Autodesk Inventor part; units mm, degrees
ref_plane "YZ Plane" through (0, 0, 0) normal (1, 0, 0) x (0, 1, 0)
ref_plane "XZ Plane" through (0, 0, 0) normal (0, 1, 0) x (-1, 0, 0)
ref_plane "XY Plane" through (0, 0, 0) normal (0, 0, 1) x (1, 0, 0)
sketch "Sketch1" plane through (0, 0, 0) normal (0, 0, 1) x (1, 0, 0)
  line L0 (-212.5, -81.5) -> (212.5, -81.5)
  line L1 (212.5, -81.5) -> (212.5, 81.5)
  line L2 (212.5, 81.5) -> (-212.5, 81.5)
  line L3 (-212.5, 81.5) -> (-212.5, -81.5)
  line L4 (-212.5, -81.5) -> (212.5, 81.5) construction
  line L5 (212.5, -81.5) -> (-212.5, 81.5) construction
  point P0 (0, 0)
  dimension "d0" = 163
  dimension "d1" = 425
extrude "Extrusion1" add sketch "Sketch1" against normal blind 335
sketch "Sketch2" plane through (-212.5, -81.5, 0) normal (0, -1, 0) x (1, 0, 0)
  line L0 (0, 0) -> (425, 0) construction
  line L1 (425, -8) -> (409.5, -8)
  line L2 (409.5, -8) -> (409.5, -28)
  line L3 (409.5, -28) -> (425, -28)
  line L4 (425, -28) -> (425, -8)
  line L5 (20, -10) -> (0, -10)
  line L6 (0, -10) -> (0, -25.5)
  line L7 (0, -25.5) -> (20, -25.5)
  line L8 (20, -25.5) -> (20, -10)
  line L9 (0, -10) -> (0, 0) construction
  line L10 (425, -8) -> (425, 0) construction
  point P0 (212.5, 0)
  dimension "d0" = 163
  dimension "d4" = 8
  dimension "d5" = 10
  dimension "d6" = 15.5
  dimension "d7" = 20
  dimension "d8" = 15.5
  dimension "d9" = 20
extrude "Extrusion2" add sketch "Sketch2" along normal blind 6
sketch "Sketch3" plane through (212.5, -81.5, 0) normal (1, 0, 0) x (0, 0, -1)
  line L0 (0, 0) -> (0, 163)
  line L1 (0, 0) -> (-5, 0)
  line L2 (-5, 0) -> (-40, 47)
  line L3 (-40, 47) -> (-90, 47)
  line L4 (-90, 47) -> (-90, 87)
  line L5 (-90, 87) -> (-69, 87)
  line L6 (-69, 93) -> (-34.909, 105.3518)
  line L7 (-69, 87) -> (-69, 93)
  arc A0 (-34.909, 105.3518) -> (-5, 148) centre (-50.3612, 148) ccw
  line L8 (-34.909, 105.3518) -> (0, 118) construction
  arc A1 (-37.8496, 44.1124) -> (-43.6003, 47) centre (-43.6003, 39.8299) ccw
  line L9 (-5, 148) -> (-5, 163)
  line L10 (-5, 163) -> (0, 163)
  dimension "d12" = 5
  dimension "d13" = 47
  dimension "d14" = 35
  dimension "d15" = 40
  dimension "d16" = 90
  dimension "d17" = 118
  dimension "d18" = 93
  dimension "d19" = 69
  dimension "d23" = 55
  dimension "d26" = 5
  dimension "d27" = 15
extrude "Extrusion3" add sketch "Sketch3" against normal blind 35
sketch "Sketch4" plane through (-212.5, -81.5, 0) normal (-1, 0, 0) x (0, 0, 1)
  line L0 (0, 0) -> (0, 163)
  line L1 (0, 0) -> (5, 0)
  line L2 (5, 0) -> (37.8496, 44.1124)
  arc A0 (43.6003, 47) -> (37.8496, 44.1124) centre (43.6003, 39.8299) ccw
  line L3 (43.6003, 47) -> (90, 47)
  line L4 (90, 47) -> (90, 87)
  line L5 (90, 87) -> (69, 87)
  line L6 (69, 87) -> (69, 93)
  line L7 (69, 93) -> (34.909, 105.3518)
  arc A1 (5, 148) -> (34.909, 105.3518) centre (50.3612, 148) ccw
  line L8 (5, 148) -> (5, 163)
  line L9 (5, 163) -> (0, 163)
  point P0 (0, 81.5)
extrude "Extrusion4" add sketch "Sketch4" against normal blind 32
sketch "Sketch5" plane through (-212.5, 81.5, -335) normal (0, 1, 0) x (1, 0, 0)
  line L0 (390, -335) -> (32, -335)
  line L1 (32, -335) -> (8, -335)
  line L2 (8, -335) -> (8, -330)
  line L3 (8, -330) -> (39, -330)
  line L4 (39, -330) -> (39, -335)
  line L5 (0, 0) -> (0, -340) construction
  point P0 (212.5, -335)
  dimension "d28" = 39
  dimension "d29" = 5
  dimension "d30" = 8
extrude "Extrusion5" add sketch "Sketch5" along normal blind 30
sketch "Sketch6" plane through (-212.5, 81.5, -335) normal (0, 1, 0) x (1, 0, 0)
  line L0 (0, 0) -> (0, -340) construction
  line L1 (390, -335) -> (39, -335)
  line L2 (212, -335) -> (212, -315)
  line L3 (212, -315) -> (240, -315)
  line L4 (240, -315) -> (240, -335)
  point P0 (212.5, -335)
  dimension "d33" = 212
  dimension "d34" = 240
  dimension "d35" = 20
extrude "Extrusion6" add sketch "Sketch6" along normal blind 5
sketch "Sketch7" plane through (0, 0, 0) normal (0, 0, 1) x (1, 0, 0)
  line L0 (177.5, 81.5) -> (27.5, 81.5)
  line L1 (32.5, 81.5) -> (32.5, 111.5)
  line L2 (-212.5, -81.5) -> (-212.5, 81.5) construction
  line L3 (102.5, 81.5) -> (102.5, 111.5)
  line L4 (32.5, 111.5) -> (102.5, 111.5)
  point P0 (0, 0)
  dimension "d38" = 245
  dimension "d39" = 315
  dimension "d40" = 30
extrude "Extrusion7" add sketch "Sketch7" against normal blind 20
sketch "Sketch8" plane through (-212.5, 81.5, -335) normal (0, 1, 0) x (1, 0, 0)
  line L0 (0, 0) -> (0, -340) construction
  line L1 (374, -315) -> (399, -315)
  line L2 (399, -315) -> (399, -320)
  line L3 (399, -320) -> (374, -320)
  line L4 (374, -320) -> (374, -315)
  line L5 (390, -335) -> (315, -335) construction
  point P0 (212.5, -335)
  dimension "d43" = 374
  dimension "d44" = 399
  dimension "d45" = 15
  dimension "d46" = 20
extrude "Extrusion8" add sketch "Sketch8" along normal blind 30
sketch "Sketch9" plane through (-212.5, 86.5, -335) normal (0, 1, 0) x (1, 0, 0)
  line L0 (240, -315) -> (212, -315)
  line L1 (240, -335) -> (240, -315)
  line L2 (212, -320) -> (240, -320)
  line L3 (212, -315) -> (212, -320)
  line L4 (8, -330) -> (8, -335) construction
  point P0 (212.5, -335)
extrude "Extrusion9" add sketch "Sketch9" along normal up to surface (25 mm away)
properties part number "IMA Battery Case Primitive"
Source: CAD feature listing. Evaluate the final solid. Frame: model axes, mm. A direction names the side the tool comes from. Give positions to 0.01 mm unless a question says otherwise; leave off trailing zeros. Write each loop counter-clockwise with the first axis right and the second up, starting at its lowest first coordinate (ties: lowest second). Pieces come first, ordered by that corner, then holes. Notation, with made-up numbers: (-17, 14.25) - (-10, 14.25) arc R11 cw to (-10, 22.25) - close; hole circle Ø5 at (-1, 78). An arc over 180 degrees is marked (long way). Write item = value, one per line. Start each with the question number.
Q1. Reachability of faces 1 (the flat face through (67, 97, -20)), 2 (the flat face through (-197, 74, 5)), 3 (the flat face through (-189, 96, -5)), 4 (the flat face through (-197, -34.5, 66)), 5 (the flat face through (174, 96, -15)) from +Z, -Z, +X, -X, +Y, -Y: full face, straight path, thin tool, end or side. Return the list, or none.
Q2. Material intervals for probe 1 along X at (y, z) = (-29, 19.5); probe 2 along Z at (x, y) = (-13.5, 1); probe 3 along Y at (x, z) = (154, -184), sorted ascending.
Q3. Pin query (flat end, axial travel): pin 1 Ø5 at (x, y) = (-207.5, -86) entering from -Z; pin 2 Ø3 at (x, z) = (97, -159.5) entering from +Y; pin 3 Ø6 at (y, z) = (95.5, -13.5) entering from -X. Return the tip coordinate at first contact, or that it passes through.
Q4. Cut plane D-D, the plane z = -172. Return loops of the section in (x, y).
Q5. Cut plane C-C, the plane y = -28. Return loops of the section in (x, z).
Q6. Cut plane A-A, the plane z = 61. Return loops of the section in (x, y), then the cut area to 3 significant figures.
Q7. Cut plane B-B, the plane x = 8.5. Return loops of the section in (y, z).
Computed values:
q1.face_1 = -Z, +X, -X, +Y
q1.face_2 = +Z, +X, -X, +Y
q1.face_3 = -Z, -X, +Y
q1.face_4 = +Z, +X, -X, -Y
q1.face_5 = +Z, +X, +Y
q2.probe_1 = -212.5 to -180.5, 177.5 to 212.5
q2.probe_2 = -335 to 0
q2.probe_3 = -81.5 to 81.5
q3.pin_1 = -25.5
q3.pin_2 = 81.5
q3.pin_3 = -0.5
q4.outline = (-212.5, -81.5) - (212.5, -81.5) - (212.5, 81.5) - (-212.5, 81.5) - close
q5.outline = (-212.5, -335) - (212.5, -335) - (212.5, 90) - (177.5, 90) - (177.5, 0) - (-180.5, 0) - (-180.5, 90) - (-212.5, 90) - close
q6.outline = (-212.5, -34.5) - (-180.5, -34.5) - (-180.5, 14.4) - (-212.5, 14.4) - close; (177.5, -34.5) - (212.5, -34.5) - (212.5, 14.4) - (177.5, 14.4) - close
q6.area = 3,280 mm²
q7.outline = (-81.5, -335) - (81.5, -335) - (81.5, -20) - (111.5, -20) - (111.5, -15) - (86.5, -15) - (86.5, 0) - (-81.5, 0) - close
